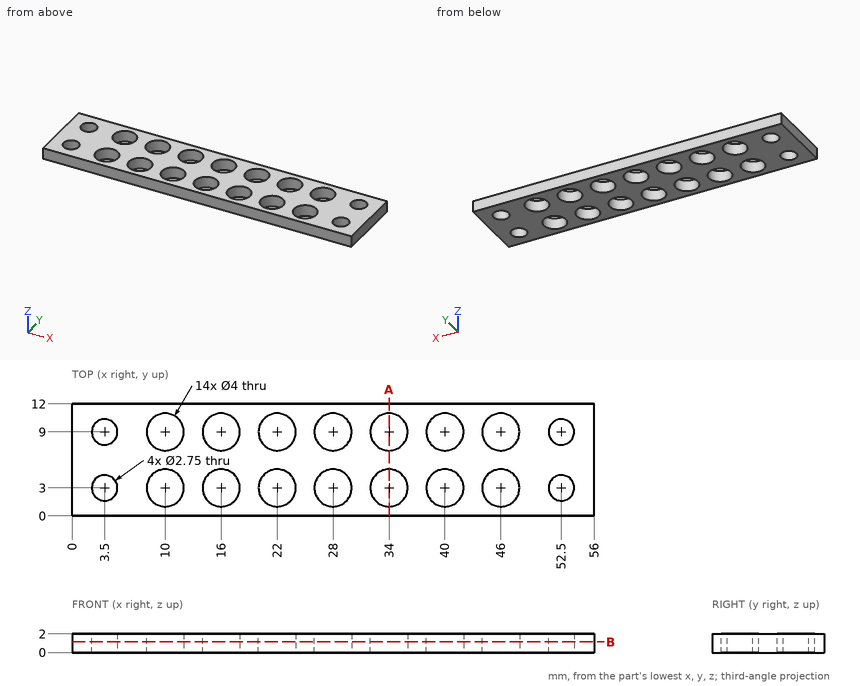
Source: three-view drawing plus pictorial views. Frame: mm from the lowest corner of the part. Give positions to 0.01 mm unless a question says otherwise; leave off trailing zeros. Order: outer loops, then holes, each group sorted by start corner. A loop starts at its lowest first (then second) coordinate and runs counter-clockwise, first axis right, second up. Notation, with made-up numbers: (42.5, -24) -> (76.5, -24) arc R14 cw to (76.5, -8) -> close; hole circle Ø5 at (77.5, 64.5). An arc over 180 degrees is marked (long way). Use a Markdown table: item, result.
Q1. Section A-A (x = 34). Return the cut outline in (y, z), and give its area (3 significant figures).
A:
| item | result |
|---|---|
| outline | (0, 0) -> (1, 0) -> (1, 2) -> (0, 2) -> close; (5, 0) -> (7, 0) -> (7, 2) -> (5, 2) -> close; (11, 0) -> (12, 0) -> (12, 2) -> (11, 2) -> close |
| area | 8.00 mm^2 |
Q2. Section B-B (z = 1.15). State how many separate pieces and enclosed holes the cut face has, and give its area (3 significant figures).
A:
| item | result |
|---|---|
| separate pieces | 1 |
| enclosed holes | 18 |
| area | 472 mm^2 |
Q3. Material intervals for line 1 (Y direction, x = 40, z = 1.25); line 2 (Y direction, x = 3.5, z = 1.45) (3 decimals), sorted ascending. Write a range as [from, to].
A:
| item | result |
|---|---|
| line 1 | [0, 1], [5, 7], [11, 12] |
| line 2 | [0, 1.625], [4.375, 7.625], [10.375, 12] |
